from build123d import *

# Parameters (mm, degrees)
CYLINDER001_R     = 2
CYLINDER001_DEPTH = 12
BOX012_W          = 10.5
BOX012_H          = 42.5
BOX012_DEPTH      = 5
CHAMFER005_SIZE   = 0.3


with BuildPart() as m4_tap:
    # Cylinder001 → Cylinder001 (new body)
    with BuildSketch(Plane.XY.offset(5)):
        Circle(CYLINDER001_R)
    extrude(amount=CYLINDER001_DEPTH)


with BuildPart() as cut:
    # Box012 → Box012 (new body)
    with BuildSketch(Plane(origin=(-5.25, -21.25, 0), x_dir=(1, 0, 0), z_dir=(0, 0, 1))):
        with Locations((5.25, 21.25)):
            Rectangle(BOX012_W, BOX012_H)
    extrude(amount=BOX012_DEPTH)

    # Chamfer005
    chamfer005_edges = [cut.edges().sort_by_distance(p)[0] for p in [
        (-5.25, -21.25, 2.5),
        (-5.25, 21.25, 2.5),
        (5.25, -21.25, 2.5),
        (5.25, 21.25, 2.5),
    ]]
    chamfer(chamfer005_edges, length=CHAMFER005_SIZE)


with BuildPart() as cut_1:
    # Chamfer005 placement: moved
    add(cut.part.moved(Location((0, 0, 10))))

    # Cut: cut M4-tap
    add(m4_tap.part, mode=Mode.SUBTRACT)


solid = cut_1.part
CAD build for the part. Positions are in the model's coordinates, mm. Coordinates: 2 decimals unless noted, no trailing zeros. Write each loop counter-clockwise with the first axis right and the second up, starting at its lowest first coordinate (ties: lowest second). Pieces come first, ordered by that corner, then holes. Notation, with made-up numbers: M -26,-26 L -15,-26 A23 cw -15,-5 Z; hole C 83.25,-25 d3. An arc over 180 degrees is marked long. Answer as a JSON object with one key per item and string values. Group by question number.
1) Saw through at A-A (y = 0). Write the cut outline in (x, z), plus the area to 3 significant figures.
2) Mould opens along X. For faces 1 (the face through (0, -21.25, 12)), 2 (the face through (0, -2, 12)), 3 (the face through (-5.25, 0, 12)) say: +X half, -X half, draft (parallel to the pull), parting line (faces both ways), or undercut.
3) Pin check, flat tip, straight feed: pin 1 Ø3 at (x, y) = (0, 0) entering from +Z. Stop position of the tip, or through.
4) Saw through at B-B (x = 0). Write the cut outline in (y, z), plus the area to 4 significant figures.
5) Wall check: line 1 (X direction, y = 0, z = 11.95); line 2 (Y direction, x = 0, z = 13.15); line 3 (X direction, y = 0.5, z = 13.65). Give the ranges that are in metal, low to high. Write a range as from..to.
6) Saw through at C-C (z = 13.05). Write the cut outline in (x, y), plus the area to 3 significant figures.
Values follow:
{
 "1": {"outline": "M -5.25,10 L -2,10 L -2,15 L -5.25,15 Z; M 2,10 L 5.25,10 L 5.25,15 L 2,15 Z", "area": "32.5 mm2"},
 "2": {"face 1": "draft", "face 2": "undercut", "face 3": "-X half"},
 "3": {"pin 1": "passes through"},
 "4": {"outline": "M -21.25,10 L -2,10 L -2,15 L -21.25,15 Z; M 2,10 L 21.25,10 L 21.25,15 L 2,15 Z", "area": "192.5 mm2"},
 "5": {"line 1": "x = -5.25..-2, 2..5.25", "line 2": "y = -21.25..-2, 2..21.25", "line 3": "x = -5.25..-1.94, 1.94..5.25"},
 "6": {"outline": "M -5.25,-20.95 L -4.95,-21.25 L 4.95,-21.25 L 5.25,-20.95 L 5.25,20.95 L 4.95,21.25 L -4.95,21.25 L -5.25,20.95 Z; hole C 0,0 d4", "area": "434 mm2"}
}
